```python
from build123d import *

# Parameters (mm, degrees)
SKETCH2_W           = 15.875
SKETCH2_H           = 7.9375
BOSS_EXTRUDE3_DEPTH = 3.175
SHELL1_T            = -1.524
FILLET1_R           = 0.254


with BuildPart() as part:
    # Sketch2 → Boss-Extrude3 (new body)
    with BuildSketch(Plane(origin=(0, 0, 0), x_dir=(1, 0, 0), z_dir=(0, 1, 0))):
        with Locations((-9.795613381, 4.754641089)):
            Rectangle(SKETCH2_W, SKETCH2_H)
    extrude(amount=BOSS_EXTRUDE3_DEPTH)

    # Shell1
    shell1_openings = [part.faces().sort_by_distance(p)[0] for p in [
        (-9.795613381, 0, -4.754641089),
    ]]
    offset(amount=SHELL1_T, openings=shell1_openings, kind=Kind.INTERSECTION)

    # Fillet1
    fillet1_edges = [part.edges().sort_by_distance(p)[0] for p in [
        (-1.858113381, 3.175, -4.754641089),
        (-9.795613381, 3.175, -8.723391089),
        (-17.733113381, 3.175, -4.754641089),
        (-17.733113381, 1.5875, -8.723391089),
        (-1.858113381, 1.5875, -8.723391089),
        (-1.858113381, 1.5875, -0.785891089),
        (-17.733113381, 1.5875, -0.785891089),
        (-9.795613381, 3.175, -0.785891089),
    ]]
    fillet(fillet1_edges, radius=FILLET1_R)


solid = part.part
```
For this review, take the finished solid that the model builds, in its own axes (mm). A direction names the side the tool comes from. Coordinates: 2 decimals unless noted, no trailing zeros. Order: outer loops, then holes, each group sorted by start corner. A loop starts at its lowest first (then second) coordinate and runs counter-clockwise, first axis right, second up. Notation, with made-up numbers: (52.25, 75) - (64.25, 75) arc R13 cw to (64.25, 90) - close; hole circle Ø1 at (83.25, -3.75). An arc over 180 degrees is marked (long way). Answer as a JSON object with one key per item and string values. Group by question number.
1. We need section C-C on x = -15.5. State the section outline as (y, z) points (3 decimals).
2. For faces 1 (the flat face through (-9.9, 0, -7.5)), 2 (the flat face through (-10, 1, -7.199)), list the 3-axis set-ups (+Z, -Z, +X, -X, +Y, -Y) from which the entire face can be reached by the end or side of a thin tool; tool diameter is ignored.
3. We need section A-A on y = 1.3. State the section outline as (x, z) points.
4. Clearance check with a flat-ended pin moving along its axis: P1, Ø2.5, axis at x = -8.5, z = -4, coming from the -Y side. State where the tip first meets the part, or that it passes through.
5. The part is to be moulded in two halves that separate along X. For faces 3 (the flat face through (-3.382, 1, -5)), 4 (the flat face through (-17.733, 1, -5)), 5 (the flat face through (-10, 1, -8.723)), say which applies: pulls with the +X half, pulls with the -X half, needs draft (parallel to the pull), parting line crosses it, or undercut.
6. We need section B-B on z = -6.5. State the section outline as (x, y) points (3 decimals).
7. For probe 1 along X at (y, z) = (0.15, -7); probe 2 along Z at (x, y) = (-14.75, 0.8); probe 3 along Y at (x, z) = (-15.5, -4.5) (3 decimals), list the stretches that pass through material, from the lowest coordinate up.
Final values:
{
 "1": {"outline": "(0, -8.723) - (2.921, -8.723) arc R0.254 ccw to (3.175, -8.469) - (3.175, -1.04) arc R0.254 ccw to (2.921, -0.786) - (0, -0.786) - (0, -2.31) - (1.651, -2.31) - (1.651, -7.199) - (0, -7.199) - close"},
 "2": {"face 1": "+Z, -Z, +X, -X, -Y", "face 2": "-Y"},
 "3": {"outline": "(-17.73, -8.47) arc R0.25 ccw to (-17.48, -8.72) - (-2.11, -8.72) arc R0.25 ccw to (-1.86, -8.47) - (-1.86, -1.04) arc R0.25 ccw to (-2.11, -0.79) - (-17.48, -0.79) arc R0.25 ccw to (-17.73, -1.04) - close; hole (-16.21, -7.2) - (-3.38, -7.2) - (-3.38, -2.31) - (-16.21, -2.31) - close"},
 "4": {"P1": "y = 1.65"},
 "5": {"face 3": "undercut", "face 4": "pulls with the -X half", "face 5": "needs draft"},
 "6": {"outline": "(-17.733, 0) - (-16.209, 0) - (-16.209, 1.651) - (-3.382, 1.651) - (-3.382, 0) - (-1.858, 0) - (-1.858, 2.921) arc R0.254 ccw to (-2.112, 3.175) - (-17.479, 3.175) arc R0.254 ccw to (-17.733, 2.921) - close"},
 "7": {"probe 1": "-17.73 to -16.21, -3.38 to -1.86", "probe 2": "-8.72 to -7.2, -2.31 to -0.79", "probe 3": "1.651 to 3.175"}
}
